from build123d import *

# Parameters (mm, degrees)
SKETCH_1_R                    = 74.5
EXTRUDE_1_DEPTH               = 14
HOLE_WIZARD_M10_1_D           = 11
HOLE_WIZARD_M10_1_CBORE_D     = 19
HOLE_WIZARD_M10_1_CBORE_DEPTH = 10.5
HOLE_WIZARD_M8_1_D            = 6.8
PATTERN_CIRCULAR_1_COUNT      = 4


with BuildPart() as part:
    # 草图1 → 凸台-拉伸1 (new body)
    with BuildSketch(Plane.XY):
        Circle(SKETCH_1_R)
    extrude(amount=EXTRUDE_1_DEPTH)

    # M10 六角头螺栓的柱形沉头孔1 (through all)
    with Locations(Plane.XY.offset(14)):
        with Locations((-33.5, 26.5), (-33.5, -53.5), (33.5, -53.5), (33.5, -13.5), (33.5, 53.5), (-33.5, 53.5)):
            CounterBoreHole(HOLE_WIZARD_M10_1_D / 2, HOLE_WIZARD_M10_1_CBORE_D / 2, HOLE_WIZARD_M10_1_CBORE_DEPTH)

    # M8 螺纹孔的螺纹孔钻头1 (through all)
    with Locations(Plane.XY.offset(14)):
        with Locations((46.669047558, 46.669047558)):
            hole_wizard_m8_1 = Hole(HOLE_WIZARD_M8_1_D / 2)

    # 阵列(圆周)1: M8 螺纹孔的螺纹孔钻头1 ×4 about axis
    pattern_circular_1_axis = Axis((0, 0, 0), (0, 0, 1))
    for i in range(1, PATTERN_CIRCULAR_1_COUNT):
        add(hole_wizard_m8_1.rotate(pattern_circular_1_axis, i * 360 / PATTERN_CIRCULAR_1_COUNT), mode=Mode.SUBTRACT)


solid = part.part
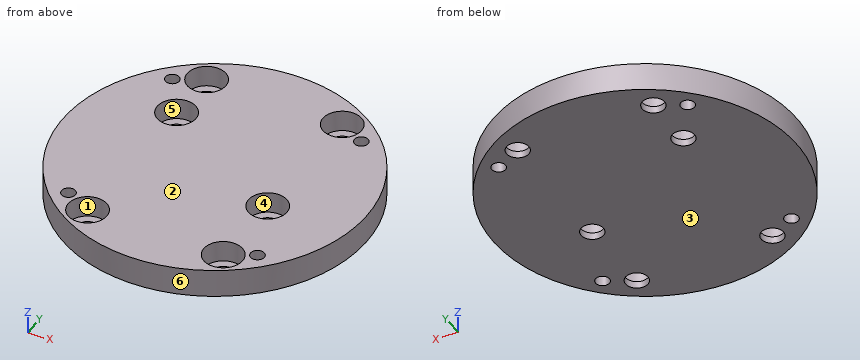
The model under review builds one solid part; all positions refer to its coordinate system, in mm. Face numbers are marked on the shaded views. A direction names the side the tool comes from. Coordinates: 2 decimals unless noted, no trailing zeros. Order: outer loops, then holes, each group sorted by start corner. A loop starts at its lowest first (then second) coordinate and runs counter-clockwise, first axis right, second up. Notation, with made-up numbers: (-13, -8.5) -> (26, -8.5) arc R24 ccw to (26, 13.5) -> close; hole circle Ø7 at (51, -13). An arc over 180 degrees is marked (long way). Answer in a Markdown table with one row per item.
(1) Consider section A-A (y = -53.5). Write out the cut boundary in (x, z), plus the area to 3 significant figures.
Answers:
| item | result |
|---|---|
| outline | (-51.85, 0) -> (-39, 0) -> (-39, 3.5) -> (-43, 3.5) -> (-43, 14) -> (-51.85, 14) -> close; (-28, 0) -> (28, 0) -> (28, 3.5) -> (24, 3.5) -> (24, 14) -> (-24, 14) -> (-24, 3.5) -> (-28, 3.5) -> close; (39, 0) -> (51.85, 0) -> (51.85, 14) -> (43, 14) -> (43, 3.5) -> (39, 3.5) -> close |
| area | 976 mm² |
(2) Consider section B-B (z = 9.25). State how many separate pieces and enclosed holes the cut face has, plus the area to 3 significant figures.
Answers:
| item | result |
|---|---|
| separate pieces | 1 |
| enclosed holes | 10 |
| area | 15,600 mm² |
(3) Consider section D-D (y = -13.5). Write out the cut boundary in (x, z).
Answers:
| item | result |
|---|---|
| outline | (-73.27, 0) -> (28, 0) -> (28, 3.5) -> (24, 3.5) -> (24, 14) -> (-73.27, 14) -> close; (39, 0) -> (73.27, 0) -> (73.27, 14) -> (43, 14) -> (43, 3.5) -> (39, 3.5) -> close |
(4) The part is to be moulded in two halves that separate along Y. For the marked faces 3, 4, 5 and 6, say which applies: +Y half, -Y half, draft (parallel to the pull), parting line (faces both ways), or undercut.
Answers:
| item | result |
|---|---|
| face 3 | draft |
| face 4 | undercut |
| face 5 | undercut |
| face 6 | parting line |
(5) Wall thickness on line 1 along X through (y, z) = (-56.5, 13.5); line 2 along Y through (x, z) = (25, 8.25); line 3 along Y through (x, z) = (-30, 6.75): over which ranges is each line inside the solid? List them lowest first.
Answers:
| item | result |
|---|---|
| line 1 | -48.56 to -42.51, -24.49 to 24.49, 42.51 to 48.56 |
| line 2 | -70.18 to -57.74, -49.26 to -17.74, -9.26 to 49.26, 57.74 to 70.18 |
| line 3 | -68.19 to -62.33, -44.67 to 17.67, 35.33 to 44.67, 62.33 to 68.19 |
(6) Insertion check: pin 1 (6.5 mm diameter, centred on x = -33.5, y = -53.5, fed in from +Z); pin 2 (3 mm diameter, centred on y = 24.5, z = 11, fed in from +X); pin 3 (4 mm diameter, centred on x = 57.5, z = 11.5, fed in from -Y); pin 4 (1 mm diameter, centred on y = -11, z = 2.5, fed in from +X). Each pin has a flat end and moves straight along its axis. Give the tip position at first contact, or say it passes through.
Answers:
| item | result |
|---|---|
| pin 1 | through |
| pin 2 | x = 70.86 |
| pin 3 | y = -49.7 |
| pin 4 | x = 73.76 |
(7) Machinability: for the marked faces 1 and 2, which of the approach directions +Z, -Z, +X, -X, +Y, -Y give a long, thin tool a straight path to every point of the face, cutting with its end or side? Answer none if there is none.
Answers:
| item | result |
|---|---|
| face 1 | +Z |
| face 2 | +Z, +X, -X, +Y, -Y |
(8) Consider section C-C (y = 26.5). Write out the cut boundary in (x, z), plus the area to 3 significant figures.
Answers:
| item | result |
|---|---|
| outline | (-69.63, 0) -> (-39, 0) -> (-39, 3.5) -> (-43, 3.5) -> (-43, 14) -> (-69.63, 14) -> close; (-28, 0) -> (69.63, 0) -> (69.63, 14) -> (-24, 14) -> (-24, 3.5) -> (-28, 3.5) -> close |
| area | 1,710 mm² |
